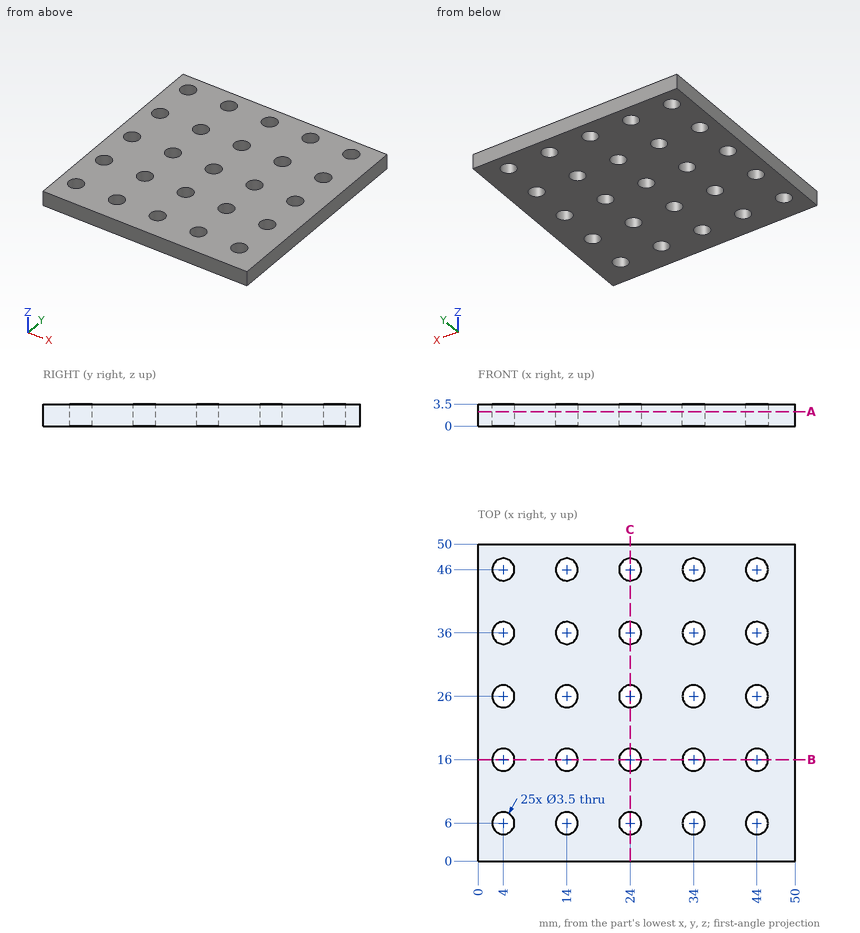
Study the drawing (mm; zero at the part's minimum x, y, z) and answer. Give positions to 0.01 mm unless a question says otherwise; leave off trailing zeros. Loops run counter-clockwise (first coordinate to the right, second up) from the corner with the lowest first, then second, coordinate; pieces in that order, holes last. Notation, with made-up numbers: (-39, 14) - (-7, 14) arc R15 cw to (-7, 20) - close; hole circle Ø3 at (33, 24). An arc over 180 degrees is marked (long way). Answer in a Markdown table with one row per item. Add a question column.
Q1. Consider line 1 along Y through (x, z) = (4, 0.9); line 2 along X through (y, z) = (25, 0.85); line 3 along Y through (x, z) = (12.5, 2.25). Determine where each line is inside the solid, lowest interval first.
Q2. The part is cut by section C-C (x = 24). Determine the outline of the cut face in (y, z).
Q3. The part is cut by section A-A (z = 2.3). State how many separate pieces and enclosed holes the cut face has, and give its area (3 significant figures).
Q4. The part is cut by section B-B (y = 16). Determine the outline of the cut face in (x, z).
Solution:
| question | item | result |
|---|---|---|
| 1 | line 1 | y = 0 to 4.25, 7.75 to 14.25, 17.75 to 24.25, 27.75 to 34.25, 37.75 to 44.25, 47.75 to 50 |
| 1 | line 2 | x = 0 to 2.56, 5.44 to 12.56, 15.44 to 22.56, 25.44 to 32.56, 35.44 to 42.56, 45.44 to 50 |
| 1 | line 3 | y = 0 to 5.1, 6.9 to 15.1, 16.9 to 25.1, 26.9 to 35.1, 36.9 to 45.1, 46.9 to 50 |
| 2 | outline | (0, 0) - (4.25, 0) - (4.25, 3.5) - (0, 3.5) - close; (7.75, 0) - (14.25, 0) - (14.25, 3.5) - (7.75, 3.5) - close; (17.75, 0) - (24.25, 0) - (24.25, 3.5) - (17.75, 3.5) - close; (27.75, 0) - (34.25, 0) - (34.25, 3.5) - (27.75, 3.5) - close; (37.75, 0) - (44.25, 0) - (44.25, 3.5) - (37.75, 3.5) - close; (47.75, 0) - (50, 0) - (50, 3.5) - (47.75, 3.5) - close |
| 3 | separate pieces | 1 |
| 3 | enclosed holes | 25 |
| 3 | area | 2,260 mm² |
| 4 | outline | (0, 0) - (2.25, 0) - (2.25, 3.5) - (0, 3.5) - close; (5.75, 0) - (12.25, 0) - (12.25, 3.5) - (5.75, 3.5) - close; (15.75, 0) - (22.25, 0) - (22.25, 3.5) - (15.75, 3.5) - close; (25.75, 0) - (32.25, 0) - (32.25, 3.5) - (25.75, 3.5) - close; (35.75, 0) - (42.25, 0) - (42.25, 3.5) - (35.75, 3.5) - close; (45.75, 0) - (50, 0) - (50, 3.5) - (45.75, 3.5) - close |
